Read the model definition and answer for the solid it produces. Units are mm, in the model's axes. A direction names the side the tool comes from. Give positions to 0.01 mm unless a question says otherwise; leave off trailing zeros. Order: outer loops, then holes, each group sorted by start corner. A loop starts at its lowest first (then second) coordinate and runs counter-clockwise, first axis right, second up.
```python
from build123d import *

# Parameters (mm, degrees)
BOSS_EXTRUDE1_DEPTH = 304.8
FILLET1_R           = 0.254


with BuildPart() as part:
    # Sketch3 → Boss-Extrude1 (new, symmetric)
    with BuildSketch(Plane.XY):
        Polygon((1.5875, 25.4), (0, 25.4), (0, 0), (25.4, 0), (25.4, 1.5875), (1.5875, 1.5875), align=None)
    extrude(amount=BOSS_EXTRUDE1_DEPTH, both=True)

    # Fillet1
    fillet1_edges = [part.edges().sort_by_distance(p)[0] for p in [
        (1.5875, 1.5875, 0),
    ]]
    fillet(fillet1_edges, radius=FILLET1_R)


solid = part.part
```
1) Given pin 1 (12 mm diameter, centred on y = 17.5, z = 68.5, fed in from +X); pin 2 (12 mm diameter, centred on x = 16, z = 108.5, fed in from +Y), each flat-ended and moving along its own axis, determine where each tip first touches the part or whether it passes through.
Final values:
pin 1: stops at x = 1.59
pin 2: stops at y = 1.59
2) The part is cut by section A-A on z = -266.5. Determine the outline of the cut face in (x, y), and give its area (3 significant figures).
Final values:
outline: (0, 0) - (25.4, 0) - (25.4, 1.59) - (1.84, 1.59) arc R0.25 cw to (1.59, 1.84) - (1.59, 25.4) - (0, 25.4) - close
area: 78.1 mm2
3) Consider L1, parallel to X at y = 2.25, z = 13.5. Determine where the line is inside the solid, lowest interval first.
Final values:
L1: x = 0 to 1.59
4) A tool of negligible diameter and unlimited length cuts with its end or side. For faces 1 (the face through (1.588, 13, 4)), 2 (the face through (1, 7, -304.8)), from which of +Z, -Z, +X, -X, +Y, -Y can it reach the whole face along a straight path? Write none if from no direction.
Final values:
face 1: +Z, -Z, +X, +Y
face 2: -Z, +X, -X, +Y, -Y
5) The part is cut by section B-B on x = 13. Determine the outline of the cut face in (y, z), and give its area (3 significant figures).
Final values:
outline: (0, -304.8) - (1.59, -304.8) - (1.59, 304.8) - (0, 304.8) - close
area: 968 mm2
